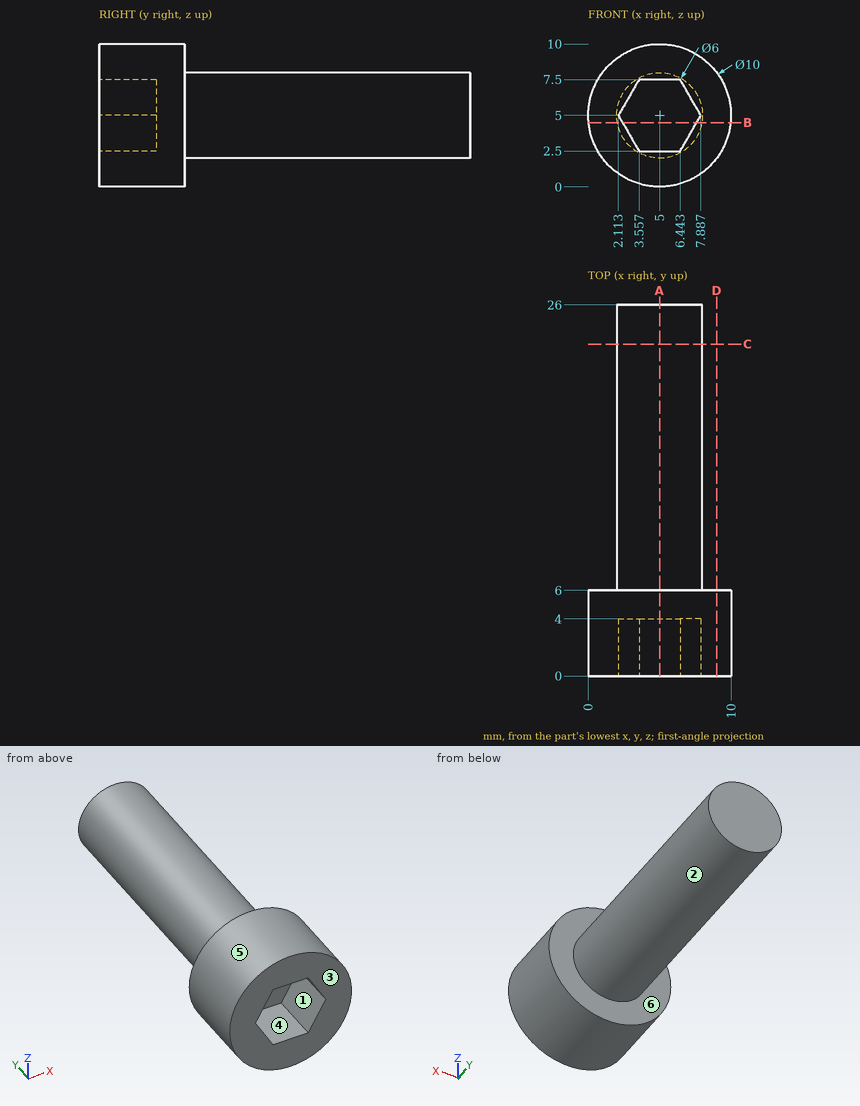
Answer from the drawing. Dimensions are ordinates in mm from the lowest x, y and z of the part. A direction names the side the tool comes from. Give positions to 0.01 mm unless a question says otherwise; leave off trailing zeros. Loops run counter-clockwise (first coordinate to the right, second up) from the corner with the lowest first, then second, coordinate; pieces in that order, holes last. Notation, with made-up numbers: M 34.5,50 L 80.5,50 A3 ccw 80.5,54 Z; hole C 2,40.5 d6. An arc over 180 degrees is marked long. One line per item, written item: value.
Q1. Flat-ended cylindrical pins translate along their axes: P1, Ø1.5, axis at x = 5.5, y = 9.5, coming from the +Z side; P2, Ø1.5, axis at x = 6, y = 13.5, coming from the -Z side; P3, Ø1.5, axis at y = 8.5, z = 3, coming from the +X side. Find the tip coordinate at first contact, or state that the pin passes through.
Working result:
P1: stops at z = 8
P2: stops at z = 2.01
P3: stops at x = 7.73
Q2. A cutting plane is placed at C-C on y = 23.25. Determine the outline of the cut face in (x, z).
Working result:
outline: C 5,5 d6
Q3. Find the intervals of material crossed by line 1 (Z direction, x = 4.75, y = 3); line 2 (Y direction, x = 4.5, z = 6.25); line 3 (Y direction, x = 2.5, z = 7), in increasing order. Write a range as from..to.
Working result:
line 1: z = 0.01..2.5, 7.5..9.99
line 2: y = 4..26
line 3: y = 0..6
Q4. A cutting plane is placed at A-A on x = 5. Determine the outline of the cut face in (y, z), then the cut area to 3 significant figures.
Working result:
outline: M 0,0 L 6,0 L 6,2 L 26,2 L 26,8 L 6,8 L 6,10 L 0,10 L 0,7.5 L 4,7.5 L 4,2.5 L 0,2.5 Z
area: 160 mm^2
Q5. For the marked faces 1, 2 and 3, determine the directions among +Z, -Z, +X, -X, +Y, -Y from which every point of the face is accessible in a straight line to the end or side of a thin tool.
Working result:
face 1: -Y
face 2: +Y
face 3: +Z, -Z, +X, -X, -Y
Q6. A cutting plane is placed at D-D on x = 9. Determine the outline of the cut face in (y, z).
Working result:
outline: M 0,2 L 6,2 L 6,8 L 0,8 Z
Q7. Determine the mould class of the marked faces 4, 5 and 6 for opening direction Z: +Z half, -Z half, draft (parallel to the pull), parting line (faces both ways), or undercut.
Working result:
face 4: undercut
face 5: parting line
face 6: draft
Q8. A cutting plane is placed at B-B on z = 4.5. Determine the outline of the cut face in (x, y) (1 decimal), then the cut area to 3 significant figures.
Working result:
outline: M 0,0 L 2.4,0 L 2.4,4 L 7.6,4 L 7.6,0 L 10,0 L 10,6 L 8,6 L 8,26 L 2,26 L 2,6 L 0,6 Z
area: 157 mm^2
